```python
from build123d import *

# Parameters (mm, degrees)
SKETCH1_W           = 43.18
SKETCH1_H           = 7.62
SKETCH1_H_2         = 3.175
SKETCH1_W_2         = 54.864
SKETCH1_H_3         = 4.191
BOSS_EXTRUDE1_DEPTH = 50.8
SKETCH2_R           = 1.4859
BOSS_EXTRUDE2_DEPTH = 5.08
FILLET1_R           = 5.08
FILLET2_R           = 5.08


with BuildPart() as part:
    # Sketch1 → Boss-Extrude1 (new body)
    with BuildSketch(Plane.XY):
        with Locations((0, 9.0805)):
            Rectangle(SKETCH1_W, SKETCH1_H)
        with Locations((0, 3.683)):
            Rectangle(SKETCH1_W, SKETCH1_H_2)
        Rectangle(SKETCH1_W_2, SKETCH1_H_3)
    extrude(amount=BOSS_EXTRUDE1_DEPTH)

    # Sketch2 → Boss-Extrude2 (add)
    with BuildSketch(Plane(origin=(0, 12.8905, 0), x_dir=(1, 0, 0), z_dir=(0, 1, 0))):
        with Locations((-18.288, -7.112)):
            Circle(SKETCH2_R)
        with Locations((18.288, -7.112)):
            Circle(SKETCH2_R)
        with Locations((18.288, -43.688)):
            Circle(SKETCH2_R)
        with Locations((-18.288, -43.688)):
            Circle(SKETCH2_R)
    extrude(amount=BOSS_EXTRUDE2_DEPTH)

    # Fillet1
    fillet1_edges = [part.edges().sort_by_distance(p)[0] for p in [
        (21.59, 7.493, 0),
        (-21.59, 7.493, 0),
        (21.59, 7.493, 50.8),
        (-21.59, 7.493, 50.8),
    ]]
    fillet(fillet1_edges, radius=FILLET1_R)

    # Fillet2
    fillet2_edges = [part.edges().sort_by_distance(p)[0] for p in [
        (27.432, 0, 0),
        (-27.432, 0, 0),
        (-27.432, 0, 50.8),
        (27.432, 0, 50.8),
    ]]
    fillet(fillet2_edges, radius=FILLET2_R)


solid = part.part
```
Here's how the part is built. I have some questions about the finished solid (model axes, mm). A direction names the side the tool comes from. Round coordinates to 2 decimals unless told otherwise and drop trailing zeros. Loops run counter-clockwise (first coordinate to the right, second up) from the corner with the lowest first, then second, coordinate; pieces in that order, holes last.
1. Suppose I cut it at C-C, the plane x = -19. Please give me the cut outline in (y, z).
Answers:
outline: (-2.1, 0) - (2.1, 0) - (2.1, 0.65) - (12.89, 0.65) - (12.89, 5.81) - (17.97, 5.81) - (17.97, 8.42) - (12.89, 8.42) - (12.89, 42.38) - (17.97, 42.38) - (17.97, 44.99) - (12.89, 44.99) - (12.89, 50.15) - (2.1, 50.15) - (2.1, 50.8) - (-2.1, 50.8) - close
2. Thinking about a two-plate mould opening in Z: for faces 1 (the face through (21.59, 7, 25)), 2 (the face through (19.66, 15.39, 44.26)), 3 (the face through (-16.915, 15.395, 44.257)), 4 (the face through (0, 6, 0)), which applies, released by +Z, released by -Z, zero draft, split by the parting line, or undercut?
Answers:
face 1: zero draft
face 2: undercut
face 3: undercut
face 4: released by -Z
3. For faces 5 (the face through (-21.59, 8, 25)), 6 (the face through (-20.141, 7.417, 1.528)), 7 (the face through (20.062, 7.569, 49.351)), which set-ups out of +Z, -Z, +X, -X, +Y, -Y let a thin tool reach every point of the face, with its end or its side?
Answers:
face 5: +Z, -Z, -X, +Y
face 6: -Z, -X, +Y
face 7: +Z, +X, +Y
4. Will these pins go through, and if not, where does the flat tip stop? pin 1 (6 mm diameter, centred on y = 10, z = 15, fed in from +X); pin 2 (3.5 mm diameter, centred on x = 20.5, z = 17.5, fed in from +Y); pin 3 (1.5 mm diameter, centred on x = -14, y = 14.5, fed in from +Z).
Answers:
pin 1: stops at x = 21.59
pin 2: stops at y = 12.89
pin 3: passes through
5. Suppose I cut it at D-D, the plane y = 15.5. Please give me the cut outline in (x, z), and give its area (3 significant figures).
Answers:
outline: circle Ø2.97 at (-18.29, 7.11); circle Ø2.97 at (-18.29, 43.69); circle Ø2.97 at (18.29, 7.11); circle Ø2.97 at (18.29, 43.69)
area: 27.7 mm2
6. Suppose I cut it at A-A, the plane z = 11. Please give me the cut outline in (x, y), and give its area (3 significant figures).
Answers:
outline: (-27.43, -2.1) - (27.43, -2.1) - (27.43, 2.1) - (21.59, 2.1) - (21.59, 12.89) - (-21.59, 12.89) - (-21.59, 2.1) - (-27.43, 2.1) - close
area: 696 mm2
7. Suppose I cut it at B-B, the plane y = 7.5. Please give me the cut outline in (x, z), and give its area (3 significant figures).
Answers:
outline: (-21.59, 5.08) arc R5.08 ccw to (-16.51, 0) - (16.51, 0) arc R5.08 ccw to (21.59, 5.08) - (21.59, 45.72) arc R5.08 ccw to (16.51, 50.8) - (-16.51, 50.8) arc R5.08 ccw to (-21.59, 45.72) - close
area: 2,170 mm2
8. If I drill on probe 1 along Z at (x, y) = (18.5, 14.5); probe 2 along Y at (x, z) = (-13, 7); probe 3 along X at (y, z) = (2.5, 42.5), over which ranges is the centre line in solid material (lowest first)?
Answers:
probe 1: z = 5.64 to 8.58, 42.22 to 45.16
probe 2: y = -2.1 to 12.89
probe 3: x = -21.59 to 21.59
